```python
from build123d import *

# Parameters (mm, degrees)
F0_W     = 10.375
F0_H     = 5.7
F0_W_2   = 4.8
F0_H_2   = 4.3
F1_DEPTH = 1
F2_W     = 0.2
F2_H     = 5.7
F3_DEPTH = 1


with BuildPart() as f1:
    # F0 (on Right) → F1 (new body)
    with BuildSketch(Plane.YZ):
        with BuildLine():
            Line((-49.5, 0), (0, 0))
            ThreePointArc((0, 0), (1.86, 8.3), (0, 16.6))
            Line((0, 16.6), (-49.5, 16.6))
            ThreePointArc((-49.5, 16.6), (-51.36, 8.3), (-49.5, 0))
        make_face()
        with Locations((-43.9125, 3.25)):
            Rectangle(F0_W, F0_H, mode=Mode.SUBTRACT)
        with Locations((-32.9375, 3.25)):
            Rectangle(F0_W, F0_H, mode=Mode.SUBTRACT)
        with Locations((-24.75, 3.25)):
            Rectangle(F0_W_2, F0_H, mode=Mode.SUBTRACT)
        with Locations((-16.5625, 3.25)):
            Rectangle(F0_W, F0_H, mode=Mode.SUBTRACT)
        with Locations((-5.5875, 3.25)):
            Rectangle(F0_W, F0_H, mode=Mode.SUBTRACT)
        with Locations((-43.9125, 13.95)):
            Rectangle(F0_W, F0_H_2, mode=Mode.SUBTRACT)
        with Locations((-32.9375, 13.95)):
            Rectangle(F0_W, F0_H_2, mode=Mode.SUBTRACT)
        with Locations((-24.75, 13.95)):
            Rectangle(F0_W_2, F0_H_2, mode=Mode.SUBTRACT)
        with Locations((-16.5625, 13.95)):
            Rectangle(F0_W, F0_H_2, mode=Mode.SUBTRACT)
        with Locations((-5.5875, 13.95)):
            Rectangle(F0_W, F0_H_2, mode=Mode.SUBTRACT)
    extrude(amount=F1_DEPTH)

    # F2 (on face) → F3 (cut, through all)
    with BuildSketch(Plane.YZ.offset(1)):
        with Locations((-49.1, 8.95)):
            Rectangle(F2_W, F2_H)
        with Locations((-38.425, 8.95)):
            Rectangle(F2_W, F2_H)
        with Locations((-27.45, 8.95)):
            Rectangle(F2_W, F2_H)
        with Locations((-22.05, 8.95)):
            Rectangle(F2_W, F2_H)
        with Locations((-11.075, 8.95)):
            Rectangle(F2_W, F2_H)
        with Locations((-0.4, 8.95)):
            Rectangle(F2_W, F2_H)
    extrude(amount=-F3_DEPTH, mode=Mode.SUBTRACT)


solid = f1.part
```
Verification items for the finished model (mm, model axes). Round coordinates to 2 decimals unless told otherwise and drop trailing zeros. Order: outer loops, then holes, each group sorted by start corner. A loop starts at its lowest first (then second) coordinate and runs counter-clockwise, first axis right, second up.
1) Cross-section at B-B, the plane z = 2. Record the cut outline in (x, y) (3 decimals).
Geometry says:
outline: (0, -50.311) - (1, -50.311) - (1, -49.1) - (0, -49.1) - close; (0, -38.725) - (1, -38.725) - (1, -38.125) - (0, -38.125) - close; (0, -27.75) - (1, -27.75) - (1, -27.15) - (0, -27.15) - close; (0, -22.35) - (1, -22.35) - (1, -21.75) - (0, -21.75) - close; (0, -11.375) - (1, -11.375) - (1, -10.775) - (0, -10.775) - close; (0, -0.4) - (1, -0.4) - (1, 0.811) - (0, 0.811) - close
2) Cross-section at C-C, the plane z = 6.75. Record the cut outline in (x, y) (3 decimals).
Geometry says:
outline: (0, -51.298) - (1, -51.298) - (1, -49.2) - (0, -49.2) - close; (0, -49) - (1, -49) - (1, -38.525) - (0, -38.525) - close; (0, -38.325) - (1, -38.325) - (1, -27.55) - (0, -27.55) - close; (0, -27.35) - (1, -27.35) - (1, -22.15) - (0, -22.15) - close; (0, -21.95) - (1, -21.95) - (1, -11.175) - (0, -11.175) - close; (0, -10.975) - (1, -10.975) - (1, -0.5) - (0, -0.5) - close; (0, -0.3) - (1, -0.3) - (1, 1.798) - (0, 1.798) - close
3) Depth check by flat-ended pin: pin 1 (0.5 mm diameter, centred on x = 0.5, z = 7.5, fed in from +Y). Enter the tip coordinate at first touch or a pass-through.
Geometry says:
pin 1: stops at y = 1.85
4) Cross-section at A-A, the plane y = -39.5. Record the cut outline in (x, z).
Geometry says:
outline: (0, 0) - (1, 0) - (1, 0.4) - (0, 0.4) - close; (0, 6.1) - (1, 6.1) - (1, 11.8) - (0, 11.8) - close; (0, 16.1) - (1, 16.1) - (1, 16.6) - (0, 16.6) - close
5) Cross-section at D-D, the plane x = 0.2. Give the number of separate pieces and of enclosed holes in the cut face, plus the area to 3 significant figures.
Geometry says:
separate pieces: 1
enclosed holes: 12
area: 393 mm2
6) Draft check along Y on faces 1 (the flat face through (1, -25, 8)), 2 (the flat face through (0.5, -22.35, 13.9)). Enter one of: +Y half, -Y half, draft (parallel to the pull), parting line (faces both ways), or undercut.
Geometry says:
face 1: draft
face 2: undercut
7) Material ranges on line 1 (Z direction, x = 0.15, y = -15); line 2 (Y direction, x = 0.9, z = 13.5) (3 decimals); line 3 (Y direction, x = 0.5, z = 12.5) (3 decimals), recorded low to high.
Geometry says:
line 1: z = 0 to 0.4, 6.1 to 11.8, 16.1 to 16.6
line 2: y = -50.652 to -49.1, -38.725 to -38.125, -27.75 to -27.15, -22.35 to -21.75, -11.375 to -10.775, -0.4 to 1.152
line 3: y = -50.901 to -49.1, -38.725 to -38.125, -27.75 to -27.15, -22.35 to -21.75, -11.375 to -10.775, -0.4 to 1.401
